Source: three-view drawing plus pictorial views. Frame: mm from the lowest corner of the part. Give positions to 0.01 mm unless a question says otherwise; leave off trailing zeros. Loops run counter-clockwise (first coordinate to the right, second up) from the corner with the lowest first, then second, coordinate; pieces in that order, holes last.
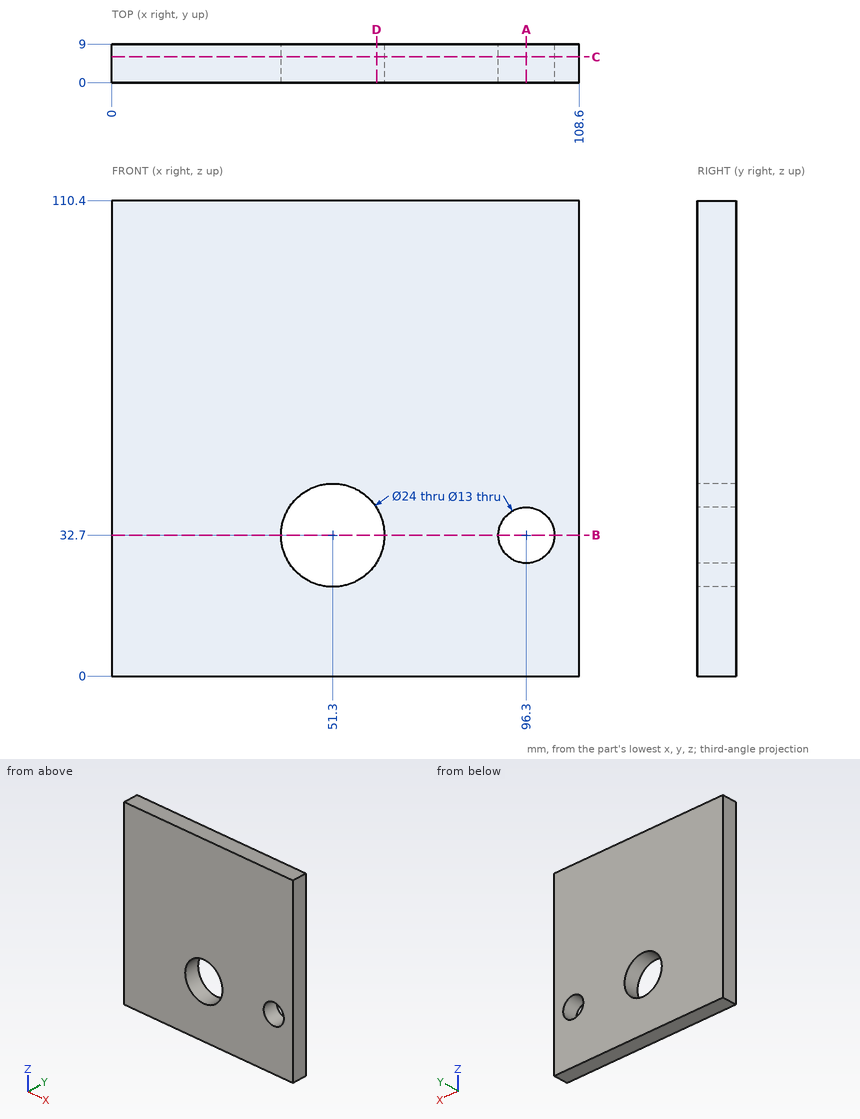
1) Cut plane D-D (x = 61.5). Return loops of the section in (y, z).
Checks:
outline: (0, 0) - (9, 0) - (9, 26.38) - (0, 26.38) - close; (0, 39.02) - (9, 39.02) - (9, 110.4) - (0, 110.4) - close
2) Cut plane C-C (y = 6). Return loops of the section in (x, z).
Checks:
outline: (0, 0) - (108.6, 0) - (108.6, 110.4) - (0, 110.4) - close; hole circle Ø24 at (51.3, 32.7); hole circle Ø13 at (96.3, 32.7)
3) Ray query, probe 1 along X at (y, z) = (2, 32.5); probe 2 along Z at (x, y) = (96.3, 4); probe 3 along X at (y, z) = (2, 22). Return the intervals inside material, ascending.
Checks:
probe 1: x = 0 to 39.3, 63.3 to 89.8, 102.8 to 108.6
probe 2: z = 0 to 26.2, 39.2 to 110.4
probe 3: x = 0 to 45.87, 56.73 to 108.6
4) Contact query for a flat-ended pin moving along its axis: P1, Ø11.5, axis at x = 96.3, z = 32.7, coming from the +Y side. Output: stop coordinate, or through.
Checks:
P1: passes through
5) Cut plane B-B (z = 32.7). Return loops of the section in (x, y).
Checks:
outline: (0, 0) - (39.3, 0) - (39.3, 9) - (0, 9) - close; (63.3, 0) - (89.8, 0) - (89.8, 9) - (63.3, 9) - close; (102.8, 0) - (108.6, 0) - (108.6, 9) - (102.8, 9) - close
6) Cut plane A-A (x = 96.3). Return loops of the section in (y, z), and give its area (3 significant figures).
Checks:
outline: (0, 0) - (9, 0) - (9, 26.2) - (0, 26.2) - close; (0, 39.2) - (9, 39.2) - (9, 110.4) - (0, 110.4) - close
area: 877 mm2
